```python
from build123d import *

# Parameters (mm, degrees)
SKETCH_R               = 1.5
PAD_DEPTH              = 1.5
SKETCH001_W            = 7.6
SKETCH001_H            = 5.4
PAD001_DEPTH           = 5
SKETCH002_R            = 0.75
POCKET_DEPTH           = 5
LINEARPATTERN_COUNT    = 20
LINEARPATTERN_PITCH    = 2.631579
SKETCH003_W            = 5.8
SKETCH003_H            = 23.5
PAD002_DEPTH           = 3.6
SKETCH004_W            = 1
SKETCH004_H            = 4.803365
PAD003_DEPTH           = 0.1
LINEARPATTERN001_COUNT = 8
LINEARPATTERN001_PITCH = 2


with BuildPart() as part:
    # Sketch → Pad (new body)
    with BuildSketch(Plane.XY):
        with BuildLine():
            ThreePointArc((-29, 28.300075), (-31.474874, 27.274949), (-32.5, 24.800075))
            Line((-32.5, -24.800075), (-32.5, 24.800075))
            ThreePointArc((-32.5, -24.800075), (-31.474874, -27.274949), (-29, -28.300075))
            Line((29, -28.300075), (-29, -28.300075))
            ThreePointArc((29, -28.300075), (31.474874, -27.274949), (32.5, -24.800075))
            Line((32.5, 24.8), (32.5, -24.800075))
            ThreePointArc((32.5, 24.8), (31.482971, 27.26675), (29.02294, 28.299925))
            Line((25.02294, 28.300075), (29.02294, 28.299925))
            Line((22.820979, 25.968397), (25.02294, 28.300075))
            Line((19.017574, 25.968397), (22.820979, 25.968397))
            Line((16.815613, 28.300075), (19.017574, 25.968397))
            Line((-29, 28.300075), (16.815613, 28.300075))
        make_face()
        with Locations((-29, 24.800075)):
            Circle(SKETCH_R, mode=Mode.SUBTRACT)
        with Locations((29, 24.8)):
            Circle(SKETCH_R, mode=Mode.SUBTRACT)
        with Locations((29, -24.800075)):
            Circle(SKETCH_R, mode=Mode.SUBTRACT)
        with Locations((-29, -24.800075)):
            Circle(SKETCH_R, mode=Mode.SUBTRACT)
    extrude(amount=PAD_DEPTH)

    # Sketch001 → Pad001 (join)
    with BuildSketch(Plane.XY):
        with Locations((-21.3, 25.600075)):
            Rectangle(SKETCH001_W, SKETCH001_H)
    extrude(amount=PAD001_DEPTH)

    # Sketch002 → Pocket (cut)
    with BuildSketch(Plane.XY):
        with Locations((-24.571527, -23.530075)):
            Circle(SKETCH002_R)
        with Locations((-24.571527, -26.070075)):
            Circle(SKETCH002_R)
    pocket = extrude(amount=POCKET_DEPTH, mode=Mode.SUBTRACT)

    # LinearPattern: Pocket ×20
    with Locations(*[(i * LINEARPATTERN_PITCH, 0, 0) for i in range(1, LINEARPATTERN_COUNT)]):
        add(pocket, mode=Mode.SUBTRACT)

    # Sketch003 → Pad002 (join)
    with BuildSketch(Plane.XY):
        with Locations((29.6, -5.550075)):
            Rectangle(SKETCH003_W, SKETCH003_H)
    extrude(amount=PAD002_DEPTH)

    # Sketch004 (on Face66 of Pad002) → Pad003 (join)
    with BuildSketch(Plane(origin=(0, 0, 0), x_dir=(1, 0, 0), z_dir=(0, 0, -1))):
        with Locations((-6.72, -22.001758)):
            Rectangle(SKETCH004_W, SKETCH004_H)
    pad003 = extrude(amount=PAD003_DEPTH)

    # LinearPattern001: Pad003 ×8
    with Locations(*[(i * LINEARPATTERN001_PITCH, 0, 0) for i in range(1, LINEARPATTERN001_COUNT)]):
        add(pad003)


solid = part.part
```
Can you work these out from the model? Positions are in its coordinate system, mm. A direction names the side the tool comes from. Give positions to 0.01 mm unless a question says otherwise; leave off trailing zeros. Order: outer loops, then holes, each group sorted by start corner. A loop starts at its lowest first (then second) coordinate and runs counter-clockwise, first axis right, second up. Notation, with made-up numbers: M 7.25,41 L 31.25,41 A8 cw 31.25,47 Z; hole C 10.5,85.25 d8. An arc over 180 degrees is marked long. One line per item, written item: value.
1) Please list where these lines run through material, in increasing order: line 1 along Y through (x, z) = (9.5, 1.4); line 2 along Z through (x, y) = (4.5, -0.5); line 3 along Y through (x, z) = (6.5, 0.6).
Answer sheet:
line 1: y = -28.3 to -26.81, -25.33 to -24.27, -22.79 to 28.3
line 2: z = 0 to 1.5
line 3: y = -28.3 to -26.62, -25.52 to -24.08, -22.98 to 28.3
2) I want a section at B-B, the plane y = -10.5. List the corners of the cut face in (x, z) for me, plus the area to 3 significant figures.
Answer sheet:
outline: M -32.5,0 L 32.5,0 L 32.5,3.6 L 26.7,3.6 L 26.7,1.5 L -32.5,1.5 Z
area: 110 mm^2
3) I want a section at C-C, the plane y = 17. List the corners of the cut face in (x, z) for me.
Answer sheet:
outline: M -32.5,0 L 32.5,0 L 32.5,1.5 L -32.5,1.5 Z
4) On a 3-axis mill with a long thin cutter (end or side, diameter ignored), from which of +Z, -Z, +X, -X, +Y, -Y can I reach the whole of each face in a straight line? I mean faces 3 (the face through (16.981, -23.023, 0.74)), 4 (the face through (-17.5, 26, 3)). Say none if no direction works.
Answer sheet:
face 3: +Z, -Z
face 4: +Z, +X, +Y, -Y
5) I want a section at A-A, the plane z = 2.65. List the corners of the cut face in (x, y) for me, plus the area to 3 significant figures.
Answer sheet:
outline: M -25.1,22.9 L -17.5,22.9 L -17.5,28.3 L -25.1,28.3 Z; M 26.7,-17.3 L 32.5,-17.3 L 32.5,6.2 L 26.7,6.2 Z
area: 177 mm^2
6) For P1, Ø1.7, axis at x = 20.17, y = -23.53, coming from the -Z side; P2, Ø0.6, axis at x = 28.5, z = 3, coming from the +Y side; P3, Ø1.7, axis at x = 7.01, y = -26.07, coming from the +Z side, each with a flat end and sliding along its axis, tell me the tip position at first contact or that it passes through.
Answer sheet:
P1: stops at z = 0
P2: stops at y = 6.2
P3: stops at z = 1.5
7) We'd pull the mould along X, two halves only. Please class faces 1 (the face through (16.94, -26.53, 0.74)), 2 (the face through (31.51, 27.24, 0.74)): released by +X, released by -X, zero draft, split by the parting line, or undercut.
Answer sheet:
face 1: undercut
face 2: released by +X
